Part print with two shaded views. Sizes in mm from the minimum x, y, z corner. A direction names the side the tool comes from. Coordinates: 2 decimals unless noted, no trailing zeros. Loops run counter-clockwise (first coordinate to the right, second up) from the corner with the lowest first, then second, coordinate; pieces in that order, holes last. Notation, with made-up numbers: (46.25, -27.5) -> (94.25, -27.5) arc R20 ccw to (94.25, 5.5) -> close; hole circle Ø2 at (28, 67.5). An arc over 180 degrees is marked (long way). Answer as a JSON object with one key per item and string values. Group by question number.
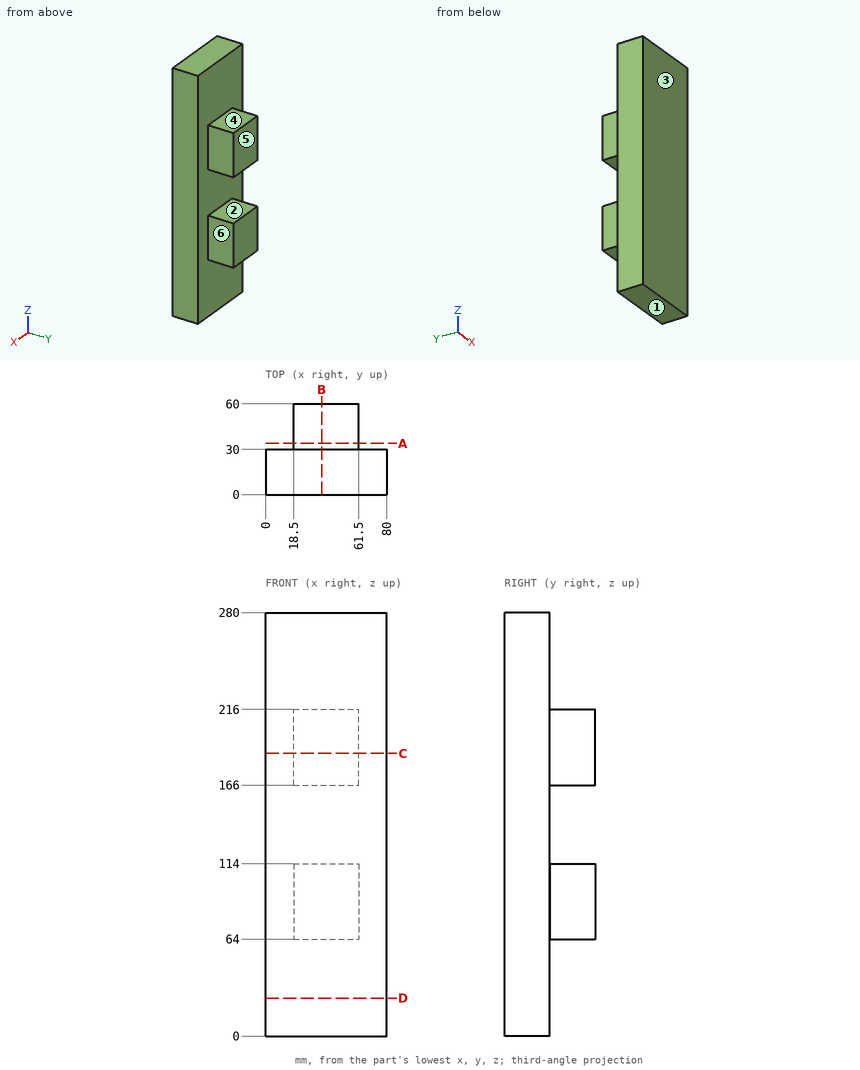
Item 1: 3-axis set-ups, long thin cutter, end or side, ignore diameter. For the marked faces 4, 5 and 6: which of +Z, -Z, +X, -X, +Y, -Y reach the whole face in a straight line?
Item 2: Drill centre lines: L1, parallel to Z at x = 38, y = 53.5; L2, parallel to Y at x = 53.5, z = 239.5. Where is each one in solid material? Low to high.
Item 3: Band-saw the part on D-D, the plane z = 25. List the corners of the cut face in (x, y), and give its area (3 significant figures).
Item 4: Pull direction Z, two halves, no side cores. Call the marked faces 1, 2 and 3: +Z half, -Z half, draft (parallel to the pull), parting line (faces both ways), or undercut.
Item 5: Band-saw the part on A-A, the plane y = 34. List the corners of the cut face in (x, z), and give its area (3 significant figures).
Item 6: Band-saw the part on C-C, the plane z = 187. List the corners of the cut face in (x, y).
Item 7: Flat gauge pins, fed straight in: P1, Ø24, axis at x = 41.5, y = 49, coming from the +Z side; P2, Ø15, axis at y = 47, z = 185.5, coming from the -X side; P3, Ø8, axis at x = 55, y = 48.5, coming from the -Z side; P4, Ø10, axis at x = 13, y = 40.5, coming from the -Z side. Where does each tip first touch, or does it go through?
Item 8: Band-saw the part on B-B, the plane x = 37. List the corners of the cut face in (y, z).
Reply:
{
 "1": {"face 4": "+Z, +X, -X, +Y", "face 5": "+Z, -Z, +X, -X, +Y", "face 6": "+Z, -Z, +X, +Y"},
 "2": {"L1": "64 to 114, 166 to 216", "L2": "0 to 30"},
 "3": {"outline": "(0, 0) -> (80, 0) -> (80, 30) -> (0, 30) -> close", "area": "2,400 mm²"},
 "4": {"face 1": "-Z half", "face 2": "undercut", "face 3": "draft"},
 "5": {"outline": "(18.5, 64) -> (61.5, 64) -> (61.5, 114) -> (18.5, 114) -> close; (18.5, 166) -> (61.5, 166) -> (61.5, 216) -> (18.5, 216) -> close", "area": "4,300 mm²"},
 "6": {"outline": "(0, 0) -> (80, 0) -> (80, 30) -> (61.5, 30) -> (61.5, 60) -> (18.5, 60) -> (18.5, 30) -> (0, 30) -> close"},
 "7": {"P1": "z = 216", "P2": "x = 18.5", "P3": "z = 64", "P4": "through"},
 "8": {"outline": "(0, 0) -> (30, 0) -> (30, 64) -> (60, 64) -> (60, 114) -> (30, 114) -> (30, 166) -> (60, 166) -> (60, 216) -> (30, 216) -> (30, 280) -> (0, 280) -> close"}
}
